```python
from build123d import *

# Parameters (mm, degrees)
SKETCH1_W           = 500
SKETCH1_H           = 500
BOSS_EXTRUDE1_DEPTH = 2.9972
SKETCH2_OUTSIDE_W   = 643.422
SKETCH2_OUTSIDE_H   = 643.422
CUT_EXTRUDE1_DEPTH  = 708.113133245


with BuildPart() as part:
    # Sketch1 → Boss-Extrude1 (new body)
    with BuildSketch(Plane(origin=(0, 0, 0), x_dir=(1, 0, 0), z_dir=(0, 1, 0))):
        with Locations((250, -250)):
            Rectangle(SKETCH1_W, SKETCH1_H)
    extrude(amount=BOSS_EXTRUDE1_DEPTH)

    # Sketch2 outside → Cut-Extrude1 (cut, through all)
    with BuildSketch(Plane(origin=(0, 2.9972, 0), x_dir=(1, 0, 0), z_dir=(0, 1, 0))):
        with Locations((250, -250)):
            Rectangle(SKETCH2_OUTSIDE_W, SKETCH2_OUTSIDE_H)
        Polygon((315.903157035, 0), (436.747635081, -264.516499207), (374.133645972, -327.130488316), (62.613989109, -327.130488316), (0, -264.516499207), (120.844478046, 0), align=None, mode=Mode.SUBTRACT)
    extrude(amount=-CUT_EXTRUDE1_DEPTH, mode=Mode.SUBTRACT)


solid = part.part
```
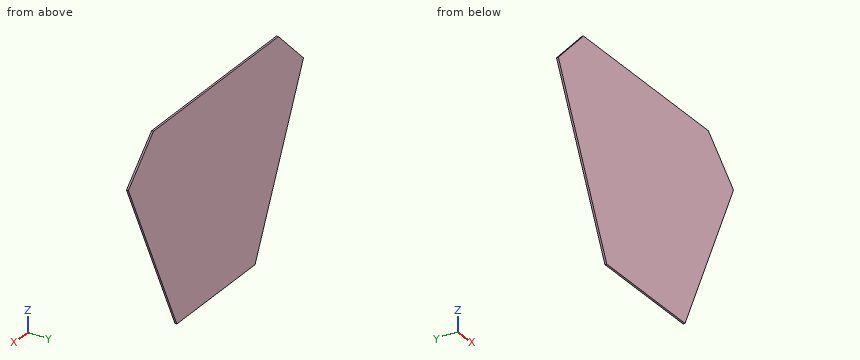
CAD build for the part. Positions are in the model's coordinates, mm. Round coordinates to 2 decimals unless told otherwise and drop trailing zeros. Write each loop counter-clockwise with the first axis right and the second up, starting at its lowest first coordinate (ties: lowest second). Pieces come first, ordered by that corner, then holes. Notation, with made-up numbers: (59.5, 14) - (90.5, 14) arc R9 ccw to (90.5, 28) - close; hole circle Ø3 at (0.25, 37). An arc over 180 degrees is marked (long way). Write item = value, one per line. Start each with the question number.
Q1. Probe L1, parallel to Z at x = 33, y = 2.7; L2, parallel to X at y = 2.4, z = 278; L3, parallel to X at y = 0.75, z = 115. List the from-to ranges inside material, lowest first. Write a range as from..to.
Q2. Band-saw the part on B-B (z = 284.5). Give the cut face in (x, y).
Q3. Band-saw the part on A-A (y = 2.4). Give the cut face in (x, z).
Q4. Band-saw the part on C-C (z = 187). Give the cut face in (x, y), then the cut area to 3 significant figures.
Answers below:
q1.L1 = 192.28..297.52
q1.L2 = 13.48..423.26
q1.L3 = 68.31..368.44
q2.outline = (19.98, 0) - (416.76, 0) - (416.76, 3) - (19.98, 3) - close
q3.outline = (0, 264.52) - (120.84, 0) - (315.9, 0) - (436.75, 264.52) - (374.13, 327.13) - (62.61, 327.13) - close
q4.outline = (35.41, 0) - (401.33, 0) - (401.33, 3) - (35.41, 3) - close
q4.area = 1,100 mm2
